from build123d import *

# Parameters (mm, degrees)
EXTRUDE_DEPTH = 25
FILLET016_R   = 2
FILLET017_R   = 0.5


with BuildPart() as part:
    # Sketch → Extrude (new body)
    with BuildSketch(Plane.XZ):
        Polygon((10.846248, 101.514289), (8.846248, 99.514289), (68.846248, 99.514289), (66.846248, 101.514289), align=None)
    extrude(amount=EXTRUDE_DEPTH)


with BuildPart() as part_1:
    # Extrude placement: moved
    add(part.part.moved(Location((0.5, -6.5, -11.5))))

    # Fillet016
    fillet016_edges = [part_1.edges().sort_by_distance(p)[0] for p in [
        (10.346248, -6.5, 89.014289),
        (68.346248, -6.5, 89.014289),
    ]]
    fillet(fillet016_edges, radius=FILLET016_R)

    # Fillet017
    fillet017_edges = [part_1.edges().sort_by_distance(p)[0] for p in [
        (9.346248, -20, 88.014289),
        (69.346248, -20, 88.014289),
    ]]
    fillet(fillet017_edges, radius=FILLET017_R)


with BuildPart() as part_2:
    # Fillet017 placement: moved
    add(part_1.part.moved(Location((-0.5, 4.5, -0.26))))


solid = part_2.part
Could you check a few things on this model? Use its own coordinates, in mm. Give positions to 0.01 mm unless a question says otherwise; leave off trailing zeros. Order: outer loops, then holes, each group sorted by start corner. A loop starts at its lowest first (then second) coordinate and runs counter-clockwise, first axis right, second up.
Item 1: I need wall thicknesses on line 1 (X direction, y = -9.5, z = 88.3); line 2 (X direction, y = -23.25, z = 89.2); line 3 (Y direction, x = 50.5, z = 88). Which ranges of each line are inside material? Lowest first, please.
Item 2: I'm going to push a flat-ended pin straight in: pin 1 (1 mm diameter, centred on y = -8, z = 89.5, fed in from -X). Where does the tip first touch, or does it pass through?
Item 3: If we section it at A-A, the plane y = -8.25: Write out the boundary of the cut face in (x, z), plus the area to 3 significant figures.
Values:
1. line 1: x = 9.56 to 68.14
1. line 2: x = 10.29 to 67.4
1. line 3: y = -27 to -2.07
2. pin 1: stops at x = 10.09
3. outline: (9.7, 88.61) arc R0.5 ccw to (10.05, 87.75) - (67.64, 87.75) arc R0.5 ccw to (67.99, 88.61) - (66.85, 89.75) - (10.85, 89.75) - close
3. area: 115 mm2
